from build123d import *

# Parameters (mm, degrees)
SKETCH1_R           = 1
SKETCH1_R_2         = 1.5
BOSS_EXTRUDE1_DEPTH = 5
SKETCH2_R           = 5
CUT_EXTRUDE1_DEPTH  = 5
SKETCH3_W           = 1.4355807
SKETCH3_H           = 6.545274718
SKETCH3_W_2         = 3.269456696
SKETCH3_H_2         = 6.030331239
CUT_EXTRUDE2_DEPTH  = 5
SKETCH4_W           = 3.74989662
SKETCH4_H           = 42
BOSS_EXTRUDE2_DEPTH = 5
FILLET1_R           = 1


with BuildPart() as part:
    # Sketch1 → Boss-Extrude1 (new body)
    with BuildSketch(Plane.XY):
        with BuildLine():
            Line((19.25, -21), (14.5, -21))
            Line((14.5, -21), (14.5, -16))
            Line((14.5, -16), (13.407179423, -16))
            Line((13.407179423, -16), (9.949944321, -16))
            ThreePointArc((9.949944321, -16), (6.076960974, -15.491376746), (2.466629547, -14))
            ThreePointArc((2.466629547, -14), (-4.754033308, -11.017246508), (-12.5, -10))
            ThreePointArc((-12.5, -10), (-22.5, 0), (-12.5, 10))
            ThreePointArc((-12.5, 10), (-4.754033308, 11.017246508), (2.466629547, 14))
            ThreePointArc((2.466629547, 14), (6.076960974, 15.491376746), (9.949944321, 16))
            Line((9.949944321, 16), (13.407179423, 16))
            Line((13.407179423, 16), (14.5, 16))
            Line((14.5, 16), (14.5, 21))
            Line((14.5, 21), (19.25, 21))
            ThreePointArc((19.25, 21), (19.426776695, 20.926776695), (19.5, 20.75))
            Line((19.5, 20.75), (19.5, 16.25))
            ThreePointArc((19.5, 16.25), (19.573223305, 16.073223305), (19.75, 16))
            Line((19.75, 16), (22.25, 16))
            ThreePointArc((22.25, 16), (22.426776695, 15.926776695), (22.5, 15.75))
            Line((22.5, 15.75), (22.5, -15.75))
            ThreePointArc((22.5, -15.75), (22.426776695, -15.926776695), (22.25, -16))
            Line((22.25, -16), (19.75, -16))
            ThreePointArc((19.75, -16), (19.573223305, -16.073223305), (19.5, -16.25))
            Line((19.5, -16.25), (19.5, -20.75))
            ThreePointArc((19.5, -20.75), (19.426776695, -20.926776695), (19.25, -21))
        make_face()
        with Locations((-19.5, -0.062454575)):
            Circle(SKETCH1_R, mode=Mode.SUBTRACT)
        with Locations((-12.562454575, 7)):
            Circle(SKETCH1_R, mode=Mode.SUBTRACT)
        with Locations((-5.5, 0.062454575)):
            Circle(SKETCH1_R, mode=Mode.SUBTRACT)
        with Locations((-12.5, 0)):
            Circle(SKETCH1_R_2, mode=Mode.SUBTRACT)
        with Locations((-12.437545425, -7)):
            Circle(SKETCH1_R, mode=Mode.SUBTRACT)
    extrude(amount=BOSS_EXTRUDE1_DEPTH)

    # Sketch2 → Cut-Extrude1 (cut)
    with BuildSketch(Plane(origin=(0, 0, 0), x_dir=(-1, 0, 0), z_dir=(0, 0, -1))):
        with Locations((12.5, 0)):
            Circle(SKETCH2_R)
    extrude(amount=-CUT_EXTRUDE1_DEPTH, mode=Mode.SUBTRACT)

    # Sketch3 → Cut-Extrude2 (cut)
    with BuildSketch(Plane(origin=(0, 0, 0), x_dir=(-1, 0, 0), z_dir=(0, 0, -1))):
        with Locations((-20.21779035, 19.272637359)):
            Rectangle(SKETCH3_W, SKETCH3_H)
        with Locations((-21.134728348, -19.01516562)):
            Rectangle(SKETCH3_W_2, SKETCH3_H_2)
    extrude(amount=-CUT_EXTRUDE2_DEPTH, mode=Mode.SUBTRACT)

    # Sketch4 → Boss-Extrude2 (add)
    with BuildSketch(Plane(origin=(0, 0, 0), x_dir=(-1, 0, 0), z_dir=(0, 0, -1))):
        with Locations((-17.62505169, 0)):
            Rectangle(SKETCH4_W, SKETCH4_H)
    extrude(amount=-BOSS_EXTRUDE2_DEPTH)

    # Fillet1
    fillet1_edges = [part.edges().sort_by_distance(p)[0] for p in [
        (19.5, -21, 2.5),
        (19.5, 21, 2.5),
        (14.5, 21, 2.5),
        (14.5, -21, 2.5),
    ]]
    fillet(fillet1_edges, radius=FILLET1_R)


solid = part.part
Verification items for the finished model (mm, model axes). A direction names the side the tool comes from. Give positions to 0.01 mm unless a question says otherwise; leave off trailing zeros. Write each loop counter-clockwise with the first axis right and the second up, starting at its lowest first coordinate (ties: lowest second). Pieces come first, ordered by that corner, then holes.
(1) Material ranges on line 1 (Y direction, x = -12.5, z = 1.05); line 2 (Y direction, x = 21, z = 0.6); line 3 (Y direction, x = -12, z = 4.3), recorded low to high.
(2) Cross-section at D-D (x = 13). Enter the section's corners in (y, z).
(3) Cross-section at C-C (z = 2.6). Enter the section's corners in (x, y).
(4) Gauge pin test, flat ends, axial feed: pin 1 (1.4 mm diameter, centred on x = 21.5, z = 2, fed in from +Y); pin 2 (1.4 mm diameter, centred on x = 13, z = 3.5, fed in from -Y); pin 3 (3 mm diameter, centred on x = 20.5, z = 3.5, fed in from -Y). Record the tip position at first contact, or that the pin passes through.
(5) Cross-section at B-B (x = -16). Enter the section's corners in (y, z), plus the area to 3 significant figures.
(6) Mould release check, pull along X, two halves, no side actions. Record for faces 1 (the face through (19.5, 18, 2)), 2 (the face through (-20.5, 0, 2.5)), 3 (the face through (-4.86, 10.99, 2.46)): +X half, -X half, draft (parallel to the pull), parting line (faces both ways), or undercut.
(7) Cross-section at A-A (y = 2). Enter the section's corners in (x, z), plus the area to 3 significant figures.
(8) Access from +Z, -Z, +X, -X, +Y, -Y to the whole of each face (thin tool, end or side, straight path). Record for faces 4 (the face through (22.5, 0, 2)), 5 (the face through (19.5, -18, 2)), 6 (the face through (14.5, -18, 2)), 7 (the face through (21, 16, 2)), 8 (the face through (12, 16, 2)).
Worked out:
1. line 1: y = -10 to -8, -6 to -5, 5 to 6, 8 to 10
1. line 2: y = -16 to 16
1. line 3: y = -10 to -7.9, -6.1 to -4.97, 4.97 to 6.17, 7.83 to 10
2. outline: (-16, 0) - (16, 0) - (16, 5) - (-16, 5) - close
3. outline: (-12.5, -10) arc R30 cw to (2.47, -14) arc R15 ccw to (9.95, -16) - (14.5, -16) - (14.5, -20) arc R1 ccw to (15.5, -21) - (18.5, -21) arc R1 ccw to (19.5, -20) - (19.5, -16) - (22.25, -16) arc R0.25 ccw to (22.5, -15.75) - (22.5, 15.75) arc R0.25 ccw to (22.25, 16) - (19.5, 16) - (19.5, 20) arc R1 ccw to (18.5, 21) - (15.5, 21) arc R1 ccw to (14.5, 20) - (14.5, 16) - (9.95, 16) arc R15 ccw to (2.47, 14) arc R30 cw to (-12.5, 10) arc R10 ccw to start; hole circle Ø2 at (-19.5, -0.06); hole circle Ø10 at (-12.5, 0); hole circle Ø2 at (-12.56, 7); hole circle Ø2 at (-12.44, -7); hole circle Ø2 at (-5.5, 0.06)
4. pin 1: stops at y = 16
4. pin 2: stops at y = -16
4. pin 3: stops at y = -20.87
5. outline: (-9.37, 0) - (-3.57, 0) - (-3.57, 5) - (-9.37, 5) - close; (3.57, 0) - (9.37, 0) - (9.37, 5) - (3.57, 5) - close
5. area: 58.0 mm2
6. face 1: +X half
6. face 2: undercut
6. face 3: -X half
7. outline: (-22.3, 0) - (-17.08, 0) - (-17.08, 5) - (-22.3, 5) - close; (-7.92, 0) - (22.5, 0) - (22.5, 5) - (-7.92, 5) - close
7. area: 178 mm2
8. face 4: +Z, -Z, +X, +Y, -Y
8. face 5: +Z, -Z, +X, -Y
8. face 6: +Z, -Z, -X, -Y
8. face 7: +Z, -Z, +X, +Y
8. face 8: +Z, -Z, -X, +Y
